```python
from build123d import *

# Parameters (mm, degrees)
CYLINDER001_R           = 56
CYLINDER001_DEPTH       = 5
CYLINDER001_PITCH_ANGLE = 90
SKETCH002_R             = 5
PAD001_DEPTH            = 10
PAD001_DEPTH_BACK       = 875


with BuildPart() as flange_for_rod001:
    # Cylinder001 → Cylinder001 (new body)
    with BuildSketch(Plane.XY):
        Circle(CYLINDER001_R)
    extrude(amount=CYLINDER001_DEPTH)


with BuildPart() as flange_for_rod001_1:
    # Cylinder001 pitch: moved
    add(flange_for_rod001.part.rotate(Axis((0, 0, 0), (0, 1, 0)), CYLINDER001_PITCH_ANGLE))


with BuildPart() as flange_for_rod001_2:
    # Cylinder001 placement: moved
    add(flange_for_rod001_1.part)


with BuildPart() as rod_flange001:
    # Sketch002 → Pad001 (new body, two sides)
    with BuildSketch(Plane.YZ) as pad001_sk:
        Circle(SKETCH002_R)
    extrude(amount=PAD001_DEPTH)
    extrude(pad001_sk.sketch, amount=-PAD001_DEPTH_BACK)

    # Fusion001: union Flange_for_Rod001
    add(flange_for_rod001_2.part)


with BuildPart() as rod_flange001_1:
    # Fusion001 placement: moved
    add(rod_flange001.part.moved(Location((250, 0, 0))))


solid = rod_flange001_1.part
```
The model under review builds one solid part; all positions refer to its coordinate system, in mm. Round coordinates to 2 decimals unless told otherwise and drop trailing zeros. Loops run counter-clockwise (first coordinate to the right, second up) from the corner with the lowest first, then second, coordinate; pieces in that order, holes last. Notation, with made-up numbers: (52, 38.5) - (56, 38.5) arc R21 ccw to (56, 66.5) - close; hole circle Ø8 at (-32.5, 35.5). An arc over 180 degrees is marked (long way). Use a Markdown table: item, result. Add a question column.
Q1. Add section A-A (z = 27.5). State the section outline as (x, y) points.
Q2. Insertion check: pin 1 Ø12 at (y, z) = (-25.5, -8) entering from -X; pin 2 Ø2 at (x, z) = (-397, -7) entering from -Y; pin 3 Ø12 at (y, z) = (17.5, 13.5) entering from +X. Each pin has a flat end and moves straight along its axis. Give the tip position at first contact, or say it passes through.
Q3. Add section C-C (y = -30). State the section outline as (x, z) points.
Q4. For probe 1 along X at (y, z) = (12, -2); probe 2 along Y at (x, z) = (30.5, -2); probe 3 along Z at (x, y) = (216, -4), list the stretches that pass through material, from the lowest coordinate up.
Q5. Add section B-B (x = -137). State the section outline as (y, z) points, plus the area to 3 significant figures.
Worked answers:
| question | item | result |
|---|---|---|
| 1 | outline | (250, -48.78) - (255, -48.78) - (255, 48.78) - (250, 48.78) - close |
| 2 | pin 1 | x = 250 |
| 2 | pin 2 | through |
| 2 | pin 3 | x = 255 |
| 3 | outline | (250, -47.29) - (255, -47.29) - (255, 47.29) - (250, 47.29) - close |
| 4 | probe 1 | 250 to 255 |
| 4 | probe 2 | -4.58 to 4.58 |
| 4 | probe 3 | -3 to 3 |
| 5 | outline | circle Ø10 at (0, 0) |
| 5 | area | 78.5 mm² |
